from build123d import *

# Parameters (mm, degrees)
SKETCH1_W           = 120
SKETCH1_H           = 50
SKETCH1_R           = 1.5
BOSS_EXTRUDE1_DEPTH = 1.53
SKETCH2_R           = 0.5
CUT_EXTRUDE1_DEPTH  = 67.229456437
SKETCH5_R           = 0.5
CUT_EXTRUDE2_DEPTH  = 67.229456437
SKETCH6_W           = 141.050966046
SKETCH6_H           = 69.53153639
CUT_EXTRUDE4_DEPTH  = 67.229456437


with BuildPart() as part:
    # Sketch1 → Boss-Extrude1 (new body)
    with BuildSketch(Plane(origin=(0, 0, 0), x_dir=(1, 0, 0), z_dir=(0, 1, 0))):
        with Locations((0, 3)):
            Rectangle(SKETCH1_W, SKETCH1_H)
        with Locations(Location((52.5, 13, 0), (0, 0, 270))):
            Circle(SKETCH1_R, mode=Mode.SUBTRACT)
        with Locations(Location((52.5, -13, 0), (0, 0, 270))):
            Circle(SKETCH1_R, mode=Mode.SUBTRACT)
        with Locations(Location((-52.5, -13, 0), (0, 0, 270))):
            Circle(SKETCH1_R, mode=Mode.SUBTRACT)
        with Locations(Location((-52.5, 13, 0), (0, 0, 270))):
            Circle(SKETCH1_R, mode=Mode.SUBTRACT)
    extrude(amount=BOSS_EXTRUDE1_DEPTH)

    # Sketch2 → Cut-Extrude1 (cut, through all)
    with BuildSketch(Plane(origin=(0, 1.53, 0), x_dir=(1, 0, 0), z_dir=(0, 1, 0))):
        with Locations(Location((-55.54, 2.54, 0), (0, 0, 270))):
            Circle(SKETCH2_R)
        with Locations(Location((-53, 2.54, 0), (0, 0, 270))):
            Circle(SKETCH2_R)
        with Locations(Location((-50.46, 2.54, 0), (0, 0, 270))):
            Circle(SKETCH2_R)
        with Locations(Location((-55.54, -2.54, 0), (0, 0, 270))):
            Circle(SKETCH2_R)
        with Locations(Location((-53, -2.54, 0), (0, 0, 270))):
            Circle(SKETCH2_R)
        with Locations(Location((-50.46, -2.54, 0), (0, 0, 270))):
            Circle(SKETCH2_R)
        with Locations(Location((-29.54, 2.54, 0), (0, 0, 270))):
            Circle(SKETCH2_R)
        with Locations(Location((-27, 2.54, 0), (0, 0, 270))):
            Circle(SKETCH2_R)
        with Locations(Location((-24.46, 2.54, 0), (0, 0, 270))):
            Circle(SKETCH2_R)
        with Locations(Location((-29.54, -2.54, 0), (0, 0, 270))):
            Circle(SKETCH2_R)
        with Locations(Location((-27, -2.54, 0), (0, 0, 270))):
            Circle(SKETCH2_R)
        with Locations(Location((-24.46, -2.54, 0), (0, 0, 270))):
            Circle(SKETCH2_R)
        with Locations(Location((-42.54, 15.54, 0), (0, 0, 270))):
            Circle(SKETCH2_R)
        with Locations(Location((-40, 15.54, 0), (0, 0, 270))):
            Circle(SKETCH2_R)
        with Locations(Location((-37.46, 15.54, 0), (0, 0, 270))):
            Circle(SKETCH2_R)
        with Locations(Location((-42.54, 10.46, 0), (0, 0, 270))):
            Circle(SKETCH2_R)
        with Locations(Location((-40, 10.46, 0), (0, 0, 270))):
            Circle(SKETCH2_R)
        with Locations(Location((-37.46, 10.46, 0), (0, 0, 270))):
            Circle(SKETCH2_R)
        with Locations(Location((-42.54, -10.46, 0), (0, 0, 270))):
            Circle(SKETCH2_R)
        with Locations(Location((-40, -10.46, 0), (0, 0, 270))):
            Circle(SKETCH2_R)
        with Locations(Location((-37.46, -10.46, 0), (0, 0, 270))):
            Circle(SKETCH2_R)
        with Locations(Location((-42.54, -15.54, 0), (0, 0, 270))):
            Circle(SKETCH2_R)
        with Locations(Location((-40, -15.54, 0), (0, 0, 270))):
            Circle(SKETCH2_R)
        with Locations(Location((-37.46, -15.54, 0), (0, 0, 270))):
            Circle(SKETCH2_R)
    cut_extrude1 = extrude(amount=-CUT_EXTRUDE1_DEPTH, mode=Mode.SUBTRACT)

    # Mirror1: Cut-Extrude1 across plane
    add(cut_extrude1.mirror(Plane(origin=(0, 0, 0), x_dir=(0, 0, 1), z_dir=(1, 0, 0))), mode=Mode.SUBTRACT)

    # Sketch5 → Cut-Extrude2 (cut, through all)
    with BuildSketch(Plane(origin=(0, 1.53, 0), x_dir=(1, 0, 0), z_dir=(0, 1, 0))):
        with Locations(Location((-2.54, 17.54, 0), (0, 0, 270))):
            Circle(SKETCH5_R)
        with Locations(Location((0, 17.54, 0), (0, 0, 270))):
            Circle(SKETCH5_R)
        with Locations(Location((2.54, 17.54, 0), (0, 0, 270))):
            Circle(SKETCH5_R)
        with Locations(Location((-2.54, 15, 0), (0, 0, 270))):
            Circle(SKETCH5_R)
        with Locations(Location((0, 15, 0), (0, 0, 270))):
            Circle(SKETCH5_R)
        with Locations(Location((2.54, 15, 0), (0, 0, 270))):
            Circle(SKETCH5_R)
    extrude(amount=-CUT_EXTRUDE2_DEPTH, mode=Mode.SUBTRACT)

    # Sketch6 → Cut-Extrude4 (cut, through all)
    with BuildSketch(Plane(origin=(0, 1.53, 0), x_dir=(1, 0, 0), z_dir=(0, 1, 0))):
        Rectangle(SKETCH6_W, SKETCH6_H)
        Polygon((-45, 28), (-60, 13), (-60, -14), (-52, -22), (-28, -22), (-24, -18), (24, -18), (28, -22), (52, -22), (60, -14), (60, 13), (45, 28), align=None, mode=Mode.SUBTRACT)
    extrude(amount=-CUT_EXTRUDE4_DEPTH, mode=Mode.SUBTRACT)


solid = part.part
Verification items for the finished model (mm, model axes). A direction names the side the tool comes from. Coordinates: 2 decimals unless noted, no trailing zeros. Order: outer loops, then holes, each group sorted by start corner. A loop starts at its lowest first (then second) coordinate and runs counter-clockwise, first axis right, second up. Notation, with made-up numbers: M -18,27 L 37,27 A10 cw 37,36 Z; hole C -25.75,72.25 d1. An arc over 180 degrees is marked long. Write each question's results on one line, items separated by ' | '.
1) Section check B-B on x = 11.5. Record the cut outline in (y, z), plus the area to 3 significant figures.
Solved:
outline: M 0,-28 L 1.53,-28 L 1.53,18 L 0,18 Z | area: 70.4 mm²
2) Section check A-A on y = 0.9. Give the number of separate pieces and of enclosed holes in the cut face, plus the area to 3 significant figures.
Solved:
separate pieces: 1 | enclosed holes: 58 | area: 5,430 mm²
3) Scan lines: line 1 along Z through (x, y) = (37.46, 0.85); line 2 along Z through (x, y) = (-29.5, 0.85); line 3 along Z through (x, y) = (6.5, 1.2). Record each from-to range of solid material in increasing order. Write a range as [from, to].
Solved:
line 1: z = [-28, -16.04], [-15.04, -10.96], [-9.96, 9.96], [10.96, 15.04], [16.04, 22] | line 2: z = [-28, -3.04], [-2.04, 2.04], [3.04, 22] | line 3: z = [-28, 18]
4) Gauge pin test, flat ends, axial feed: pin 1 Ø0.5 at (x, y) = (5, 0.5) entering from +Z; pin 2 Ø1.8 at (x, z) = (-52.5, -13) entering from -Y. Record the tip position at first contact, or that the pin passes through.
Solved:
pin 1: stops at z = 18 | pin 2: passes through
5) Release check for a two-part mould opening along Z. For faces 3 (the face through (-1, 1.53, -3)), 4 (the face through (-54, 1, 13)), 5 (the face through (-26, 1, 20)), 6 (the face through (-52, 1, -21)) record: pulls with the +Z half, pulls with the -Z half, needs draft (parallel to the pull), parting line crosses it, or undercut.
Solved:
face 3: needs draft | face 4: undercut | face 5: pulls with the +Z half | face 6: pulls with the -Z half
6) Access from +Z, -Z, +X, -X, +Y, -Y to the whole of each face (thin tool, end or side, straight path). Record for faces 1 (the face through (-54, 1, -13)), 2 (the face through (26, 1, 20)).
Solved:
face 1: +Y, -Y | face 2: +Z, +Y, -Y
